Work out the finished part from the listing and answer in its coordinate system (mm). Face numbers are marked on the shaded views. Round coordinates to 2 decimals unless told otherwise and drop trailing zeros. Write each loop counter-clockwise with the first axis right and the second up, starting at its lowest first coordinate (ties: lowest second). Pieces come first, ordered by that corner, then holes. Notation, with made-up numbers: M 32.25,-12.75 L 53.25,-12.75 A20 cw 53.25,17.25 Z; hole C 52.25,66.25 d8. An arc over 180 degrees is marked long. One line per item, written item: value. Start each with the question number.
Q1. Find section C-C (y = -1.4). Write down the section's boundary in (x, z), and give its area (3 significant figures).
Q2. Find section B-B (x = -15). Write down the section's boundary in (y, z).
Q3. Consider probe 1 along Y at (x, z) = (-10, 3.25); probe 2 along X at (y, z) = (0.45, 3); probe 3 along Y at (x, z) = (-21, 2.75). Determine where each line is inside the solid, lowest interval first.
Q4. Find section D-D (z = 5.25). Write down the section's boundary in (x, y).
Q5. Find section A-A (z = 2.5). Write down the section's boundary in (x, y), and give its area (3 significant figures).
Q6. The mould has two halves that part along X. Classify the marked faces 1, 2 and 3: released by +X, released by -X, zero draft, split by the parting line, or undercut.
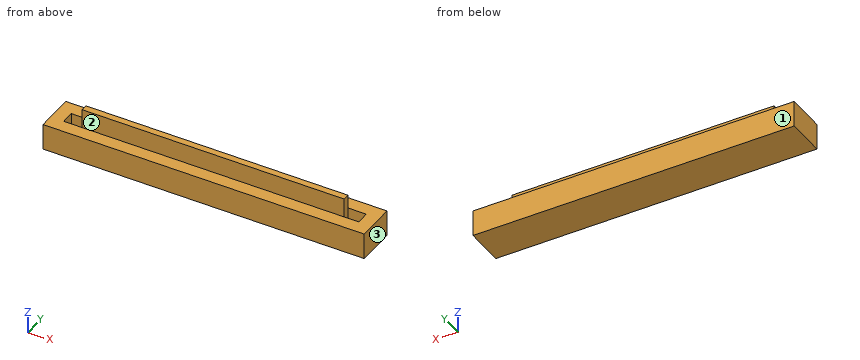
from build123d import *

# Parameters (mm, degrees)
SKETCH1_W           = 45
SKETCH1_H           = 2
BOSS_EXTRUDE1_DEPTH = 2
SKETCH1_3_W         = 49
SKETCH1_3_H         = 6
SKETCH1_3_W_2       = 45
SKETCH1_3_H_2       = 2
BOSS_EXTRUDE2_DEPTH = 4
SKETCH2_W           = 40
SKETCH2_H           = 1
BOSS_EXTRUDE3_DEPTH = 4.5


with BuildPart() as part:
    # Sketch1 → Boss-Extrude1 (new body)
    with BuildSketch(Plane.XY):
        Rectangle(SKETCH1_W, SKETCH1_H)
    extrude(amount=BOSS_EXTRUDE1_DEPTH)

    # Sketch1<3> → Boss-Extrude2 (add)
    with BuildSketch(Plane.XY):
        Rectangle(SKETCH1_3_W, SKETCH1_3_H)
        Rectangle(SKETCH1_3_W_2, SKETCH1_3_H_2, mode=Mode.SUBTRACT)
    extrude(amount=BOSS_EXTRUDE2_DEPTH)

    # Sketch2 → Boss-Extrude3 (add)
    with BuildSketch(Plane.XY.offset(2)):
        Rectangle(SKETCH2_W, SKETCH2_H)
    extrude(amount=BOSS_EXTRUDE3_DEPTH)


solid = part.part
The answers:
1. outline: M -24.5,0 L 24.5,0 L 24.5,4 L -24.5,4 Z
1. area: 196 mm2
2. outline: M -3,0 L 3,0 L 3,4 L 1,4 L 1,2 L 0.5,2 L 0.5,6.5 L -0.5,6.5 L -0.5,2 L -1,2 L -1,4 L -3,4 Z
3. probe 1: -3 to -1, -0.5 to 0.5, 1 to 3
3. probe 2: -24.5 to -22.5, -20 to 20, 22.5 to 24.5
3. probe 3: -3 to -1, 1 to 3
4. outline: M -20,-0.5 L 20,-0.5 L 20,0.5 L -20,0.5 Z
5. outline: M -24.5,-3 L 24.5,-3 L 24.5,3 L -24.5,3 Z; M -20,-0.5 L 20,-0.5 L 20,0.5 L -20,0.5 Z; hole M -22.5,-1 L 22.5,-1 L 22.5,1 L -22.5,1 Z
5. area: 244 mm2
6. face 1: zero draft
6. face 2: undercut
6. face 3: released by +X
